```python
from build123d import *

# Parameters (mm, degrees)
CROQUIS1_R              = 20
SALIENTE_EXTRUIR1_DEPTH = 10
CORTAR_EXTRUIR1_DEPTH   = 10
CROQUIS3_R              = 6.665733382
CORTAR_EXTRUIR2_DEPTH   = 10
CORTAR_EXTRUIR3_DEPTH   = 10


with BuildPart() as part:
    # Croquis1 → Saliente-Extruir1 (new body)
    with BuildSketch(Plane(origin=(0, 0, 0), x_dir=(1, 0, 0), z_dir=(0, 1, 0))):
        Circle(CROQUIS1_R)
    extrude(amount=SALIENTE_EXTRUIR1_DEPTH)

    # Croquis2 → Cortar-Extruir1 (cut)
    with BuildSketch(Plane(origin=(0, 10, 0), x_dir=(1, 0, 0), z_dir=(0, 1, 0))):
        Polygon((7.691342951, -4.440598923), (7.691342951, -9.059401077), (11.691342951, -11.368802154), (15.691342951, -9.059401077), (15.691342951, -4.440598923), (11.691342951, -2.131197846), align=None)
        Polygon((0, 8.881197846), (4, 11.190598923), (4, 15.809401077), (0, 18.118802154), (-4, 15.809401077), (-4, 11.190598923), align=None)
        Polygon((-7.691342951, -4.440598923), (-11.691342951, -2.131197846), (-15.691342951, -4.440598923), (-15.691342951, -9.059401077), (-11.691342951, -11.368802154), (-7.691342951, -9.059401077), align=None)
    extrude(amount=-CORTAR_EXTRUIR1_DEPTH, mode=Mode.SUBTRACT)

    # Croquis3 → Cortar-Extruir2 (cut)
    with BuildSketch(Plane(origin=(0, 10, 0), x_dir=(1, 0, 0), z_dir=(0, 1, 0))):
        Circle(CROQUIS3_R)
    extrude(amount=-CORTAR_EXTRUIR2_DEPTH, mode=Mode.SUBTRACT)

    # Croquis4 → Cortar-Extruir3 (cut)
    with BuildSketch(Plane(origin=(0, 10, 0), x_dir=(1, 0, 0), z_dir=(0, 1, 0))):
        Polygon((-11.691342951, 11.657477288), (-15.941342951, 9.203738644), (-15.941342951, 4.296261356), (-11.691342951, 1.842522712), (-7.441342951, 4.296261356), (-7.441342951, 9.203738644), align=None)
        Polygon((0, -18.407477288), (4.25, -15.953738644), (4.25, -11.046261356), (0, -8.592522712), (-4.25, -11.046261356), (-4.25, -15.953738644), align=None)
        Polygon((15.941342951, 4.296261356), (15.941342951, 9.203738644), (11.691342951, 11.657477288), (7.441342951, 9.203738644), (7.441342951, 4.296261356), (11.691342951, 1.842522712), align=None)
    extrude(amount=-CORTAR_EXTRUIR3_DEPTH, mode=Mode.SUBTRACT)


solid = part.part
```
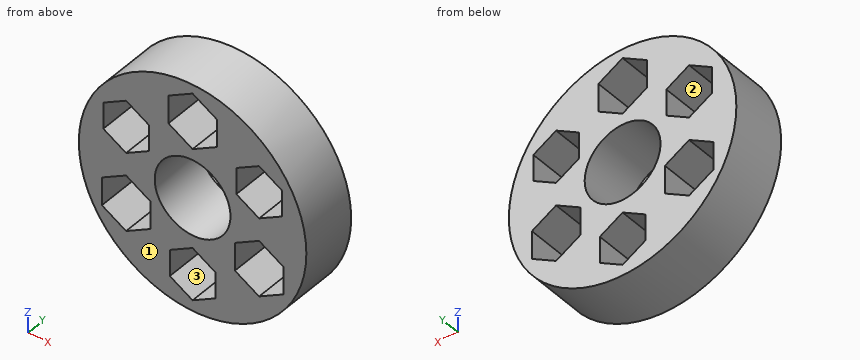
Geometry check sheet. Reference: the model listing, model coordinates, mm. Face numbers are marked on the shaded views. Coordinates: 2 decimals unless noted, no trailing zeros. Order: outer loops, then holes, each group sorted by start corner. A loop starts at its lowest first (then second) coordinate and runs counter-clockwise, first axis right, second up. Notation, with made-up numbers: (20, 83) - (40, 83) arc R15 cw to (40, 87) - close; hole circle Ø5 at (23.5, 59). An arc over 180 degrees is marked (long way). Answer as a JSON object with one key per item and string values. Group by question number.
Item 1: Scan lines: probe 1 along Z at (x, y) = (0, 6); probe 2 along X at (y, z) = (3.25, 0); probe 3 along Z at (x, y) = (2, 1.75). Record each from-to range of solid material in increasing order.
Item 2: Sectioned sample at A-A, the plane z = 0. Record the cut outline in (x, y).
Item 3: Sectioned sample at B-B, the plane x = -1.5. Record the cut outline in (y, z).
Item 4: Draft check along Z on the marked faces 1, 2 and 3. Enter one of: +Z half, -Z half, draft (parallel to the pull), parting line (faces both ways), or undercut.
Item 5: Sectioned sample at C-C, the plane x = 9. Record the cut outline in (y, z).
Item 6: Depth check by flat-ended pin: pin 1 Ø1 at (y, z) = (9, 10) entering from +X; pin 2 Ø3.5 at (y, z) = (7, 7) entering from -X; pin 3 Ø2.5 at (y, z) = (6.5, -13.5) entering from -X. Enter the tip coordinate at first touch or a pass-through.
Item 7: Sectioned sample at D-D, the plane z = -5. Record the cut outline in (x, y), and give its area (3 significant figures).
Resolved:
{
 "1": {"probe 1": "-20 to -18.12, -8.88 to -6.67, 6.67 to 8.59, 18.41 to 20", "probe 2": "-20 to -6.67, 6.67 to 20", "probe 3": "-19.9 to -16.96, -10.04 to -6.36, 6.36 to 9.75, 17.25 to 19.9"},
 "2": {"outline": "(-20, 0) - (-6.67, 0) - (-6.67, 10) - (-20, 10) - close; (6.67, 0) - (20, 0) - (20, 10) - (6.67, 10) - close"},
 "3": {"outline": "(0, -19.94) - (10, -19.94) - (10, -17.25) - (0, -17.25) - close; (0, -9.75) - (10, -9.75) - (10, -6.49) - (0, -6.49) - close; (0, 6.49) - (10, 6.49) - (10, 9.46) - (0, 9.46) - close; (0, 17.54) - (10, 17.54) - (10, 19.94) - (0, 19.94) - close"},
 "4": {"face 1": "draft", "face 2": "undercut", "face 3": "undercut"},
 "5": {"outline": "(0, -17.86) - (10, -17.86) - (10, -10.1) - (0, -10.1) - close; (0, -3.4) - (10, -3.4) - (10, 3.69) - (0, 3.69) - close; (0, 9.81) - (10, 9.81) - (10, 17.86) - (0, 17.86) - close"},
 "6": {"pin 1": "x = 17.6", "pin 2": "x = -19.3", "pin 3": "x = -15.81"},
 "7": {"outline": "(-19.36, 0) - (-15.94, 0) - (-15.94, 10) - (-19.36, 10) - close; (-7.44, 0) - (-4.41, 0) - (-4.41, 10) - (-7.44, 10) - close; (4.41, 0) - (7.44, 0) - (7.44, 10) - (4.41, 10) - close; (15.94, 0) - (19.36, 0) - (19.36, 10) - (15.94, 10) - close", "area": "129 mm^2"}
}
